Model file for the job. Use its own axes, mm. Face numbers are marked on the shaded views. A direction names the side the tool comes from. Round coordinates to 2 decimals unless told otherwise and drop trailing zeros. Order: outer loops, then holes, each group sorted by start corner. A loop starts at its lowest first (then second) coordinate and runs counter-clockwise, first axis right, second up. Notation, with made-up numbers: (4, 81.25) -> (61, 81.25) arc R27 cw to (61, 108.25) -> close; hole circle Ø4 at (-23.75, -29). An arc over 180 degrees is marked (long way). Use CSV: the item, a comma, the result in double quotes.
```python
from build123d import *

# Parameters (mm, degrees)
BOSS_EXTRUDE1_DEPTH = 69
SKETCH4_W           = 15
SKETCH4_H           = 150.1
BOSS_EXTRUDE2_DEPTH = 61.9
BOSS_EXTRUDE3_DEPTH = 20.4
FILLET1_R           = 10


with BuildPart() as part:
    # Sketch2 → Boss-Extrude1 (new body, symmetric)
    with BuildSketch(Plane(origin=(0, 0, 0), x_dir=(0, 0, -1), z_dir=(1, 0, 0))):
        with BuildLine():
            Line((-262.793626597, 0), (0, 0))
            Line((0, 0), (165.1, 0))
            Line((165.1, 0), (165.1, 81.9))
            Line((165.1, 81.9), (150.1, 81.9))
            Line((150.1, 81.9), (150.1, 20))
            Line((150.1, 20), (0, 20))
            Line((0, 20), (0, 133.7))
            Line((0, 133.7), (-115, 133.7))
            Line((-115, 133.7), (-171.193830238, 94.352656466))
            Line((-171.193830238, 94.352656466), (-262.793626597, 81.479144628))
            Line((-262.793626597, 81.479144628), (-262.793626597, 31.479144628))
            ThreePointArc((-262.793626597, 31.479144628), (-272.644060375, 15.739572314), (-262.793626597, 0))
        make_face()
    extrude(amount=BOSS_EXTRUDE1_DEPTH, both=True)

    # Sketch4 → Boss-Extrude2 (add)
    with BuildSketch(Plane(origin=(0, 20, 0), x_dir=(1, 0, 0), z_dir=(0, 1, 0))):
        with Locations((61.5, 75.05)):
            Rectangle(SKETCH4_W, SKETCH4_H)
    boss_extrude2 = extrude(amount=BOSS_EXTRUDE2_DEPTH)

    # Mirror1: Boss-Extrude2 across plane
    add(boss_extrude2.mirror(Plane(origin=(0, 0, 0), x_dir=(0, 0, 1), z_dir=(1, 0, 0))))

    # Sketch5 → Boss-Extrude3 (add)
    with BuildSketch(Plane(origin=(69, 0, 0), x_dir=(0, 0, -1), z_dir=(1, 0, 0))):
        with BuildLine():
            Line((-224.944060375, 0), (-160.344060375, 0))
            ThreePointArc((-160.344060375, 0), (-192.644060375, -32.3), (-224.944060375, 0))
        make_face()
        with BuildLine():
            Line((28.055939625, 0), (92.655939625, 0))
            ThreePointArc((92.655939625, 0), (60.355939625, -32.3), (28.055939625, 0))
        make_face()
    boss_extrude3 = extrude(amount=-BOSS_EXTRUDE3_DEPTH)

    # Mirror2: Boss-Extrude3 across plane
    add(boss_extrude3.mirror(Plane(origin=(0, 0, 0), x_dir=(0, 0, 1), z_dir=(1, 0, 0))))

    # Fillet1
    fillet1_edges = [part.edges().sort_by_distance(p)[0] for p in [
        (0, 31.479144628, 262.793626597),
        (0, 81.479144628, 262.793626597),
        (0, 94.352656466, 171.193830238),
        (0, 133.7, 115),
        (0, 133.7, 0),
    ]]
    fillet(fillet1_edges, radius=FILLET1_R)


solid = part.part
```
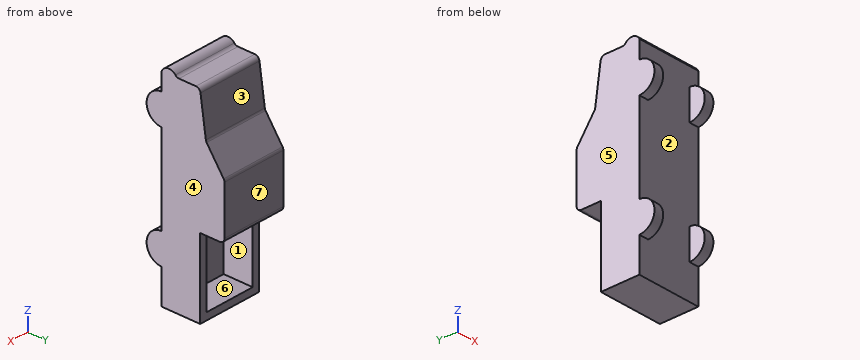
Q1. Mould opens along X. For the marked faces 4, 5, 6 and 7 say: +X half, -X half, draft (parallel to the pull), parting line (faces both ways), or undercut.
From the geometry:
face 4,"+X half"
face 5,"-X half"
face 6,"undercut"
face 7,"draft"
Q2. Cut at D-D (z = 180). Give the cut face in (x, y).
From the geometry:
outline,"(-69, -29.72) -> (-48.6, -29.72) -> (-48.6, 0) -> (48.6, 0) -> (48.6, -29.72) -> (69, -29.72) -> (69, 93.12) -> (-69, 93.12) -> close"
Q3. Pin check, flat tips, straight feed: pin 1 (1 mm diameter, centred on x = -42, z = -37, fed in from +Y); pin 2 (2 mm diameter, centred on x = 4, z = -108.5, fed in from -Y); pin 3 (10 mm diameter, centred on x = 41.5, y = -7.5, fed in from +Z). Stop position of each tip, or through.
From the geometry:
pin 1,"stops at y = 20"
pin 2,"stops at y = 0"
pin 3,"passes through"
Q4. Probe line 1 along Z through (x, y) = (26, 57.5); line 2 along X through (y, z) = (33, -57); line 3 along Y through (x, z) = (61, 67.5). List the from-to ranges inside material, lowest first.
From the geometry:
line 1,"z = -165.1 to -150.1, 0 to 262.79"
line 2,"x = -69 to -54, 54 to 69"
line 3,"y = 0 to 133.7"
Q5. Cut at B-B (y = 42.5). Give the cut face in (x, z), plus the area to 3 significant figures.
From the geometry:
outline,"(-69, -165.1) -> (69, -165.1) -> (69, 262.79) -> (-69, 262.79) -> close; hole (-54, -150.1) -> (54, -150.1) -> (54, 0) -> (-54, 0) -> close"
area,"42,800 mm²"
Q6. Which spindle directions (+Z, -Z, +X, -X, +Y, -Y) get a long thin tool onto all of the face, cutting with end or side? Do the marked faces 1, 2 and 3. Say none if no direction does.
From the geometry:
face 1,"+Y"
face 2,"-Y"
face 3,"+Z, +X, -X, +Y"
Q7. Cut at C-C (x = -5). Give the cut face in (y, z), plus the area to 3 significant figures.
From the geometry:
outline,"(0, -165.1) -> (81.9, -165.1) -> (81.9, -150.1) -> (20, -150.1) -> (20, 0) -> (123.7, 0) arc R10 ccw to (133.7, 10) -> (133.7, 111.85) arc R10 ccw to (131.89, 117.58) -> (95.73, 169.23) arc R10 cw to (94.02, 173.57) -> (82.69, 254.19) arc R10 ccw to (72.79, 262.79) -> (36.83, 262.79) arc R10 cw to (29.16, 266.38) arc R17.5 ccw to (0, 262.79) -> close"
area,"34,300 mm²"
Q8. Cut at A-A (x = -58.5). Give the cut face in (y, z).
From the geometry:
outline,"(0, -165.1) -> (81.9, -165.1) -> (81.9, 0) -> (123.7, 0) arc R10 ccw to (133.7, 10) -> (133.7, 111.85) arc R10 ccw to (131.89, 117.58) -> (95.73, 169.23) arc R10 cw to (94.02, 173.57) -> (82.69, 254.19) arc R10 ccw to (72.79, 262.79) -> (36.83, 262.79) arc R10 cw to (29.16, 266.38) arc R17.5 ccw to (0, 262.79) -> (0, 224.94) arc R32.3 ccw to (0, 160.34) -> (0, -28.06) arc R32.3 ccw to (0, -92.66) -> close"
